from build123d import *

# Parameters (mm, degrees)
PAD008_DEPTH          = 10
SKETCH025_R           = 2.6
POCKET015_DEPTH       = 73.249467
POCKET016_DEPTH       = 3.75
POLARPATTERN005_COUNT = 2
POLARPATTERN006_COUNT = 4
SKETCH026_W           = 8.15
SKETCH026_H           = 4.15
POCKET017_DEPTH       = 10


with BuildPart() as part:
    # Sketch023 → Pad008 (new body)
    with BuildSketch(Plane.XY):
        with BuildLine():
            Line((-36.624733, 5.256321), (-36.624733, -5.256321))
            ThreePointArc((-36.624733, -5.256321), (-26.162951, -26.162951), (-5.256321, -36.624733))
            Line((-5.256321, -36.624733), (5.256321, -36.624733))
            ThreePointArc((5.256321, -36.624733), (26.162951, -26.162951), (36.624733, -5.256321))
            Line((36.624733, 5.256321), (36.624733, -5.256321))
            ThreePointArc((36.624733, 5.256321), (26.162951, 26.162951), (5.256321, 36.624733))
            Line((-5.256321, 36.624733), (5.256321, 36.624733))
            ThreePointArc((-5.256321, 36.624733), (-26.162951, 26.162951), (-36.624733, 5.256321))
        make_face()
        with BuildLine():
            Line((-29.027936, -5.256321), (-29.027936, 5.256321))
            ThreePointArc((-5, 29.073184), (-20.767423, 20.951471), (-29.027936, 5.256321))
            Line((-5, 29.073184), (5, 29.073184))
            ThreePointArc((29.027936, 5.256321), (20.767423, 20.951471), (5, 29.073184))
            Line((29.027936, 5.256321), (29.027936, -5.256321))
            ThreePointArc((5.256321, -29.027936), (20.85965, -20.85965), (29.027936, -5.256321))
            Line((-5.256321, -29.027936), (5.256321, -29.027936))
            ThreePointArc((-29.027936, -5.256321), (-20.85965, -20.85965), (-5.256321, -29.027936))
        make_face(mode=Mode.SUBTRACT)
    extrude(amount=PAD008_DEPTH)

    # Sketch025 (on Face4 of Pad008) → Pocket015 (cut)
    with BuildSketch(Plane.XZ.offset(36.624733)):
        with Locations((0, 5)):
            Circle(SKETCH025_R)
    pocket015 = extrude(amount=-POCKET015_DEPTH, mode=Mode.SUBTRACT)

    # Sketch024 (on Face6 of Pad008) → Pocket016 (cut)
    with BuildSketch(Plane.YZ.offset(36.624733)):
        Polygon((4.705405, 5), (2.352702, 9.075), (-2.352702, 9.075), (-4.705405, 5), (-2.352702, 0.925), (2.352702, 0.925), align=None)
    pocket016 = extrude(amount=-POCKET016_DEPTH, mode=Mode.SUBTRACT)

    # PolarPattern005: Pocket016 ×2 about axis
    polarpattern005_axis = Axis((0, 0, 0), (0, 0, 1))
    for i in range(1, POLARPATTERN005_COUNT):
        add(pocket016.rotate(polarpattern005_axis, i * 360 / POLARPATTERN005_COUNT), mode=Mode.SUBTRACT)

    # PolarPattern006: Pocket015 ×4 about axis
    polarpattern006_axis = Axis((0, 0, 0), (0, 0, 1))
    for i in range(1, POLARPATTERN006_COUNT):
        add(pocket015.rotate(polarpattern006_axis, i * 360 / POLARPATTERN006_COUNT), mode=Mode.SUBTRACT)

    # Sketch026 (on Face5 of PolarPattern006) → Pocket017 (cut)
    with BuildSketch(Plane.XY.offset(10)):
        with Locations((0, -32.826335)):
            Rectangle(SKETCH026_W, SKETCH026_H)
        with Locations((0, 32.754596)):
            Rectangle(SKETCH026_W, SKETCH026_H)
    extrude(amount=-POCKET017_DEPTH, mode=Mode.SUBTRACT)


solid = part.part
Design review of the part built by this model. Coordinates are the model's own, in mm. A direction names the side the tool comes from. Coordinates: 2 decimals unless noted, no trailing zeros. Write each loop counter-clockwise with the first axis right and the second up, starting at its lowest first coordinate (ties: lowest second). Pieces come first, ordered by that corner, then holes. Notation, with made-up numbers: (78, 5) -> (108, 5) arc R8 cw to (108, 11) -> close; hole circle Ø3 at (0.25, -9). An arc over 180 degrees is marked (long way). Write each question's results on one line, items separated by ' | '. Start each with the question number.
(1) Clearance check with flat-ended pins moving along their axes: P1, Ø1.5, axis at x = -23.5, z = 4, coming from the +Y side; P2, Ø2, axis at y = 33, z = 6.5, coming from the +X side; P3, Ø2.5, axis at y = -1, z = 5, coming from the -X side; P4, Ø2, axis at y = -32.5, z = 6.5, coming from the +X side. State where each tip first meets the part, or that it passes through.
(2) The part is to be moulded in two halves that separate along X. For faces 1 (the face through (29.028, 2, 3)), 2 (the face through (0, -30, 0)), 3 (the face through (-25.926, 26.397, 4.93)), say which applies: pulls with the +X half, pulls with the -X half, needs draft (parallel to the pull), parting line crosses it, or undercut.
(3) Take a section at D-D on y = 16. Write out the cut boundary in (x, z).
(4) Take a section at A-A on y = 0. Write out the cut boundary in (x, z) (3 decimals).
(5) For line 1 along Y through (x, z) = (5, 8.75); line 2 along Z through (x, y) = (-32, 0); line 3 along Y through (x, z) = (16.5, 4.5), list the stretches that pass through material, from the lowest coordinate up. Write a range as from..to.
(6) Tool access review of faces 4 (the face through (-34.776, -3.546, 7.009)), 5 (the face through (-0.338, -35.775, 7.578)), 6 (the face through (-4.075, -33, 5)): name each direction out of +Z, -Z, +X, -X, +Y, -Y from which nothing blocks a thin tool from reaching the whole face with its end or side.
(7) Take a section at C-C on x = 19.5. Write out the cut boundary in (y, z), and give its area (3 significant figures).
(8) Take a section at B-B on x = 0. Give the number of separate pieces and of enclosed holes in the cut face, and give its area (3 significant figures).
Results found:
1) P1: stops at y = 29.18 | P2: stops at x = 18.57 | P3: passes through | P4: stops at x = 19.41
2) face 1: undercut | face 2: needs draft | face 3: pulls with the -X half
3) outline: (-33.36, 0) -> (-24.78, 0) -> (-24.78, 10) -> (-33.36, 10) -> close; (24.78, 0) -> (33.36, 0) -> (33.36, 10) -> (24.78, 10) -> close
4) outline: (-36.625, 0) -> (-29.028, 0) -> (-29.028, 2.4) -> (-32.875, 2.4) -> (-32.875, 0.925) -> (-36.625, 0.925) -> close; (-36.625, 9.075) -> (-32.875, 9.075) -> (-32.875, 7.6) -> (-29.028, 7.6) -> (-29.028, 10) -> (-36.625, 10) -> close; (29.028, 0) -> (36.625, 0) -> (36.625, 0.925) -> (32.875, 0.925) -> (32.875, 2.4) -> (29.028, 2.4) -> close; (29.028, 7.6) -> (32.875, 7.6) -> (32.875, 9.075) -> (36.625, 9.075) -> (36.625, 10) -> (29.028, 10) -> close
5) line 1: y = -36.62..-29.03, 29.07..36.62 | line 2: z = 0..2.4, 7.6..10 | line 3: y = -33.12..-24.45, 24.45..33.12
6) face 4: -X | face 5: +Y, -Y | face 6: +Z, -Z
7) outline: (-31.44, 0) -> (-22.14, 0) -> (-22.14, 10) -> (-31.44, 10) -> close; (22.14, 0) -> (31.44, 0) -> (31.44, 10) -> (22.14, 10) -> close | area: 186 mm2
8) separate pieces: 8 | enclosed holes: 0 | area: 32.9 mm2
